Could you check a few things on this model? Use its own coordinates, in mm. A direction names the side the tool comes from. Coordinates: 2 decimals unless noted, no trailing zeros. Loops run counter-clockwise (first coordinate to the right, second up) from the corner with the lowest first, then second, coordinate; pieces in that order, holes last.
1) For faces 4 (the face through (41, 1, 5)), 5 (the face through (1, 1, -3)), which set-ups out of +Z, -Z, +X, -X, +Y, -Y let a thin tool reach every point of the face, with its end or its side?
2) Imagine slicing it at D-D on z = -3.5. Please give me the cut outline in (x, y).
3) Imagine slicing it at B-B on x = -32.5. Please give me the cut outline in (y, z).
4) Thinking about a two-plate mould opening in X: for faces 1 (the face through (-41, 1, 5)), 2 (the face through (37.99, 1.01, -20.15)), 3 (the face through (7, 1, 6.5)), which applies, released by +X, released by -X, zero draft, split by the parting line, or undercut?
5) Imagine slicing it at C-C on z = -9. Please give me the cut outline in (x, y), plus the area to 3 significant figures.
6) If I drill on line 1 along X through (y, z) = (0.9, -3.5); line 2 along Z through (x, y) = (30, 0.3); line 3 along X through (y, z) = (0.65, -2), over which ranges is the centre line in solid material (lowest first)?
7) Will these pins go through, and if not, where does the flat tip stop? P1, Ø1.5, axis at x = 1.5, z = 10.5, coming from the -Y side; P2, Ø1, axis at x = -23.5, z = -15, coming from the +Y side.
8) Imagine slicing it at A-A on y = 1.2. Please give me the cut outline in (x, z), plus the area to 3 significant figures.
```python
from build123d import *

# Parameters (mm, degrees)
SKETCH_1_W      = 82
SKETCH_1_H      = 46
SKETCH_1_R      = 12.5
SKETCH_1_W_2    = 12.5
SKETCH_1_H_2    = 20
EXTRUDE_1_DEPTH = 2
FILLET_1_R      = 10


with BuildPart() as part:
    # 草图1 → 凸台-拉伸1 (new body)
    with BuildSketch(Plane(origin=(0, 0, 0), x_dir=(1, 0, 0), z_dir=(0, 1, 0))):
        Rectangle(SKETCH_1_W, SKETCH_1_H)
        with Locations(Location((-21.5, 3.5, 0), (0, 0, 270))):
            Circle(SKETCH_1_R, mode=Mode.SUBTRACT)
        with Locations((7.25, 3.5)):
            Rectangle(SKETCH_1_W_2, SKETCH_1_H_2, mode=Mode.SUBTRACT)
        with Locations((29.75, 3.5)):
            Rectangle(SKETCH_1_W_2, SKETCH_1_H_2, mode=Mode.SUBTRACT)
    extrude(amount=EXTRUDE_1_DEPTH)

    # 圆角1
    fillet_1_edges = [part.edges().sort_by_distance(p)[0] for p in [
        (-41, 1, -23),
        (41, 1, -23),
    ]]
    fillet(fillet_1_edges, radius=FILLET_1_R)


solid = part.part
```
Filled in:
1. face 4: +Z, -Z, +X, +Y, -Y
1. face 5: +Y, -Y
2. outline: (-41, 0) - (-34, 0) - (-34, 2) - (-41, 2) - close; (-9, 0) - (1, 0) - (1, 2) - (-9, 2) - close; (13.5, 0) - (23.5, 0) - (23.5, 2) - (13.5, 2) - close; (36, 0) - (41, 0) - (41, 2) - (36, 2) - close
3. outline: (0, -22.89) - (2, -22.89) - (2, -9.44) - (0, -9.44) - close; (0, 2.44) - (2, 2.44) - (2, 23) - (0, 23) - close
4. face 1: released by -X
4. face 2: released by +X
4. face 3: undercut
5. outline: (-41, 0) - (-32.72, 0) - (-32.72, 2) - (-41, 2) - close; (-10.28, 0) - (1, 0) - (1, 2) - (-10.28, 2) - close; (13.5, 0) - (23.5, 0) - (23.5, 2) - (13.5, 2) - close; (36, 0) - (41, 0) - (41, 2) - (36, 2) - close
5. area: 69.1 mm2
6. line 1: x = -41 to -34, -9 to 1, 13.5 to 23.5, 36 to 41
6. line 2: z = -23 to -13.5, 6.5 to 23
6. line 3: x = -41 to -33.91, -9.09 to 1, 13.5 to 23.5, 36 to 41
7. P1: stops at y = 0
7. P2: passes through
8. outline: (-41, -13) arc R10 ccw to (-31, -23) - (31, -23) arc R10 ccw to (41, -13) - (41, 23) - (-41, 23) - close; hole circle Ø25 at (-21.5, -3.5); hole (1, -13.5) - (13.5, -13.5) - (13.5, 6.5) - (1, 6.5) - close; hole (23.5, -13.5) - (36, -13.5) - (36, 6.5) - (23.5, 6.5) - close
8. area: 2,740 mm2
